```python
from build123d import *

# Parameters (mm, degrees)
ESQUISSE1_W                                       = 125
ESQUISSE1_H                                       = 6
CHANFREIN1_SIZE                                   = 1
DIAM_TRE_DU_PER_AGE_4_0_4_1_D                     = 4
DIAM_TRE_DU_PER_AGE_4_0_4_1_DEPTH                 = 11
DIAM_TRE_DU_PER_AGE_4_0_4_1_CSINK_D               = 5
DIAM_TRE_DU_PER_AGE_4_0_4_1_CSINK_ANGLE           = 90
DIAM_TRE_DU_PER_AGE_4_0_4_1_TIP                   = 1.201721238
DIAM_TRE_DU_PER_AGE_4_0_4_1_ON_FACE_2_D           = 4
DIAM_TRE_DU_PER_AGE_4_0_4_1_ON_FACE_2_DEPTH       = 11
DIAM_TRE_DU_PER_AGE_4_0_4_1_ON_FACE_2_CSINK_D     = 5
DIAM_TRE_DU_PER_AGE_4_0_4_1_ON_FACE_2_CSINK_ANGLE = 90
DIAM_TRE_DU_PER_AGE_4_0_4_1_ON_FACE_2_TIP         = 1.201721238


with BuildPart() as part:
    # Esquisse1 → Révolution1 (revolve)
    with BuildSketch(Plane.XY, mode=Mode.PRIVATE) as r_volution1_sk:
        with Locations((0, 3)):
            Rectangle(ESQUISSE1_W, ESQUISSE1_H)
    revolve(r_volution1_sk.sketch.rotate(Axis((-35.682971619, 0, 0), (1, 0, 0)), 90), axis=Axis((-35.682971619, 0, 0), (1, 0, 0)))

    # Chanfrein1
    chanfrein1_edges = [part.edges().sort_by_distance(p)[0] for p in [
        (62.5, 0, -6),
        (-62.5, 0, -6),
    ]]
    chamfer(chanfrein1_edges, length=CHANFREIN1_SIZE)

    # Diamètre du perçage Ø4.0 (4)1
    with Locations(Plane(origin=(62.5, 0, 0), x_dir=(0, 0, 1), z_dir=(1, 0, 0))):
        with Locations((0, 0)):
            CounterSinkHole(DIAM_TRE_DU_PER_AGE_4_0_4_1_D / 2, DIAM_TRE_DU_PER_AGE_4_0_4_1_CSINK_D / 2, depth=DIAM_TRE_DU_PER_AGE_4_0_4_1_DEPTH, counter_sink_angle=DIAM_TRE_DU_PER_AGE_4_0_4_1_CSINK_ANGLE)
            with Locations((0, 0, -(DIAM_TRE_DU_PER_AGE_4_0_4_1_DEPTH + DIAM_TRE_DU_PER_AGE_4_0_4_1_TIP / 2))):  # 118° drill point
                Cone(0, DIAM_TRE_DU_PER_AGE_4_0_4_1_D / 2, DIAM_TRE_DU_PER_AGE_4_0_4_1_TIP, mode=Mode.SUBTRACT)

    # Diamètre du perçage Ø4.0 (4)1 on face 2
    with Locations(Plane(origin=(-62.5, 0, 0), x_dir=(0, 0, -1), z_dir=(-1, 0, 0))):
        with Locations((0, 0)):
            CounterSinkHole(DIAM_TRE_DU_PER_AGE_4_0_4_1_ON_FACE_2_D / 2, DIAM_TRE_DU_PER_AGE_4_0_4_1_ON_FACE_2_CSINK_D / 2, depth=DIAM_TRE_DU_PER_AGE_4_0_4_1_ON_FACE_2_DEPTH, counter_sink_angle=DIAM_TRE_DU_PER_AGE_4_0_4_1_ON_FACE_2_CSINK_ANGLE)
            with Locations((0, 0, -(DIAM_TRE_DU_PER_AGE_4_0_4_1_ON_FACE_2_DEPTH + DIAM_TRE_DU_PER_AGE_4_0_4_1_ON_FACE_2_TIP / 2))):  # 118° drill point
                Cone(0, DIAM_TRE_DU_PER_AGE_4_0_4_1_ON_FACE_2_D / 2, DIAM_TRE_DU_PER_AGE_4_0_4_1_ON_FACE_2_TIP, mode=Mode.SUBTRACT)


solid = part.part
```
Check sheet for the modelled part. Datum: model origin and axes. Units: mm. A direction names the side the tool comes from. Round coordinates to 2 decimals unless told otherwise and drop trailing zeros. Loops run counter-clockwise (first coordinate to the right, second up) from the corner with the lowest first, then second, coordinate; pieces in that order, holes last. Notation, with made-up numbers: (-12, 17.25) - (-3, 17.25) arc R9 ccw to (-3, 31.25) - close; hole circle Ø8 at (57, -22). An arc over 180 degrees is marked (long way). Write item = value, one per line. Start each with the question number.
Q1. Depth check by flat-ended pin: P1, Ø6, axis at y = 4.5, z = -3.5, coming from the -X side; P2, Ø3, axis at y = 0, z = 0, coming from the +X side; P3, Ø4.5, axis at y = 0, z = 0, coming from the +X side; P4, Ø1, axis at x = -22.5, z = 4.5, coming from the -Y side. Enter the tip coordinate at first touch or a pass-through.
Q2. Access from +Z, -Z, +X, -X, +Y, -Y to the whole of each face (thin tool, end or side, straight path). Record for faces 1 (the face through (62.5, 2, -2)), 2 (the face through (57, 2, 0)).
Q3. Release check for a two-part mould opening along Y. For faces 3 (the face through (-62.5, 2, -2)), 4 (the face through (-57, 2, 0)), 5 (the face through (0.861, -1.802, 5.723)) record: pulls with the +Y half, pulls with the -Y half, needs draft (parallel to the pull), parting line crosses it, or undercut.
Q4. Thickness scan on L1, parallel to Y at x = 60.25, z = 0; L2, parallel to Y at x = -11.5, z = -0.5; L3, parallel to X at y = 0.5, z = 1.25. Record the ranges inside material, lowest first.
Q5. Section check A-A (x = 12.5). Record the boundary of the cut face in (y, z).
Derived:
q1.P1 = -62.5
q1.P2 = 51.2
q1.P3 = 62.25
q1.P4 = -4.47
q2.face_1 = +Z, -Z, +X, +Y, -Y
q2.face_2 = +X
q3.face_3 = needs draft
q3.face_4 = undercut
q3.face_5 = parting line crosses it
q4.L1 = -6 to -2, 2 to 6
q4.L2 = -5.98 to 5.98
q4.L3 = -51.11 to 51.11
q5.outline = circle Ø12 at (0, 0)
